```python
from build123d import *

# Parameters (mm, degrees)
SALIENTE_EXTRUIR1_DEPTH = 2


with BuildPart() as part:
    # Croquis1 → Saliente-Extruir1 (new body)
    with BuildSketch(Plane(origin=(0, 0, 0), x_dir=(1, 0, 0), z_dir=(0, 1, 0))):
        with BuildLine():
            Line((-41.528381643, 41.192203833), (9.471618357, 41.192203833))
            ThreePointArc((9.471618357, 41.192203833), (10.88583192, 40.606417395), (11.471618357, 39.192203833))
            Line((11.471618357, 39.192203833), (11.471618357, 2.692203833))
            ThreePointArc((11.471618357, 2.692203833), (10.88583192, 1.27799027), (9.471618357, 0.692203833))
            ThreePointArc((9.471618357, 0.692203833), (-1.488536751, -3.847641059), (-6.028381643, -14.807796167))
            ThreePointArc((-6.028381643, -14.807796167), (-6.61416808, -16.22200973), (-8.028381643, -16.807796167))
            Line((-8.028381643, -16.807796167), (-24.028381643, -16.807796167))
            ThreePointArc((-24.028381643, -16.807796167), (-25.442595205, -16.22200973), (-26.028381643, -14.807796167))
            ThreePointArc((-26.028381643, -14.807796167), (-30.568226534, -3.847641059), (-41.528381643, 0.692203833))
            ThreePointArc((-41.528381643, 0.692203833), (-42.942595205, 1.27799027), (-43.528381643, 2.692203833))
            Line((-43.528381643, 2.692203833), (-43.528381643, 39.192203833))
            ThreePointArc((-43.528381643, 39.192203833), (-42.942595205, 40.606417395), (-41.528381643, 41.192203833))
        make_face()
    extrude(amount=SALIENTE_EXTRUIR1_DEPTH)


solid = part.part
```
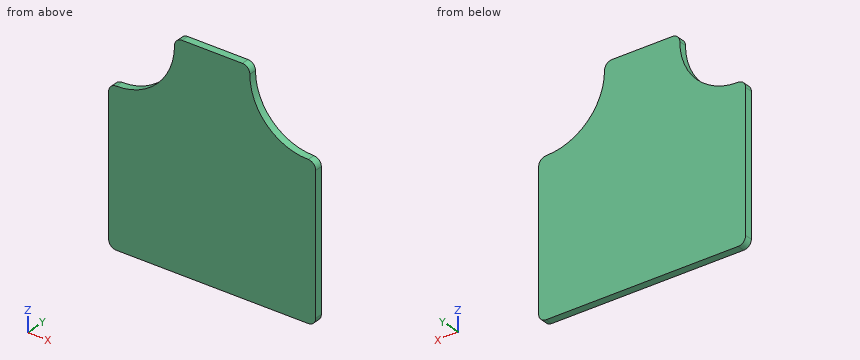
Check sheet for the modelled part. Datum: model origin and axes. Units: mm. Give positions to 0.01 mm unless a question says otherwise; leave off trailing zeros. Order: outer loops, then holes, each group sorted by start corner. A loop starts at its lowest first (then second) coordinate and runs counter-clockwise, first axis right, second up. Notation, with made-up numbers: M 54,26 L 70,26 A23 cw 70,35 Z; hole C -7.5,-25.5 d11. An arc over 180 degrees is marked long. Answer in a Markdown table with one row per item.
1) Cross-section at B-B, the plane x = -37. Enter the section's corners in (y, z).
Filled sheet:
| item | result |
|---|---|
| outline | M 0,-41.19 L 2,-41.19 L 2,-0.02 L 0,-0.02 Z |
2) Cross-section at A-A, the plane y = 0.6. Enter the section's corners in (x, z), plus the area to 3 significant figures.
Filled sheet:
| item | result |
|---|---|
| outline | M -43.53,-39.19 A2 ccw -41.53,-41.19 L 9.47,-41.19 A2 ccw 11.47,-39.19 L 11.47,-2.69 A2 ccw 9.47,-0.69 A15.5 cw -6.03,14.81 A2 ccw -8.03,16.81 L -24.03,16.81 A2 ccw -26.03,14.81 A15.5 cw -41.53,-0.69 A2 ccw -43.53,-2.69 Z |
| area | 2,680 mm2 |
3) Thickness scan on L1, parallel to Z at x = -6.5, y = 1.05; L2, parallel to X at y = 1.35, z = 4; L3, parallel to X at y = 1.4, z = 13.5. Record the ranges inside material, lowest first. Write a range as [from, to].
Filled sheet:
| item | result |
|---|---|
| L1 | z = [-41.19, 16.1] |
| L2 | x = [-30.42, -1.64] |
| L3 | x = [-26.08, -5.97] |
4) Gauge pin test, flat end, axial feed: P1, Ø1, axis at y = 1.5, z = 8.5, coming from the +X side. Record the tip position at first contact, or that the pin passes through.
Filled sheet:
| item | result |
|---|---|
| P1 | stops at x = -4.45 |
5) Cross-section at C-C, the plane z = 0. Enter the section's corners in (x, y), plus the area to 3 significant figures.
Filled sheet:
| item | result |
|---|---|
| outline | M -36.95,0 L 4.89,0 L 4.89,2 L -36.95,2 Z |
| area | 83.7 mm2 |
